Source: three-view drawing plus pictorial views. Frame: mm from the lowest corner of the part. A direction names the side the tool comes from. Give positions to 0.01 mm unless a question says otherwise; leave off trailing zeros. Loops run counter-clockwise (first coordinate to the right, second up) from the corner with the lowest first, then second, coordinate; pieces in that order, holes last.
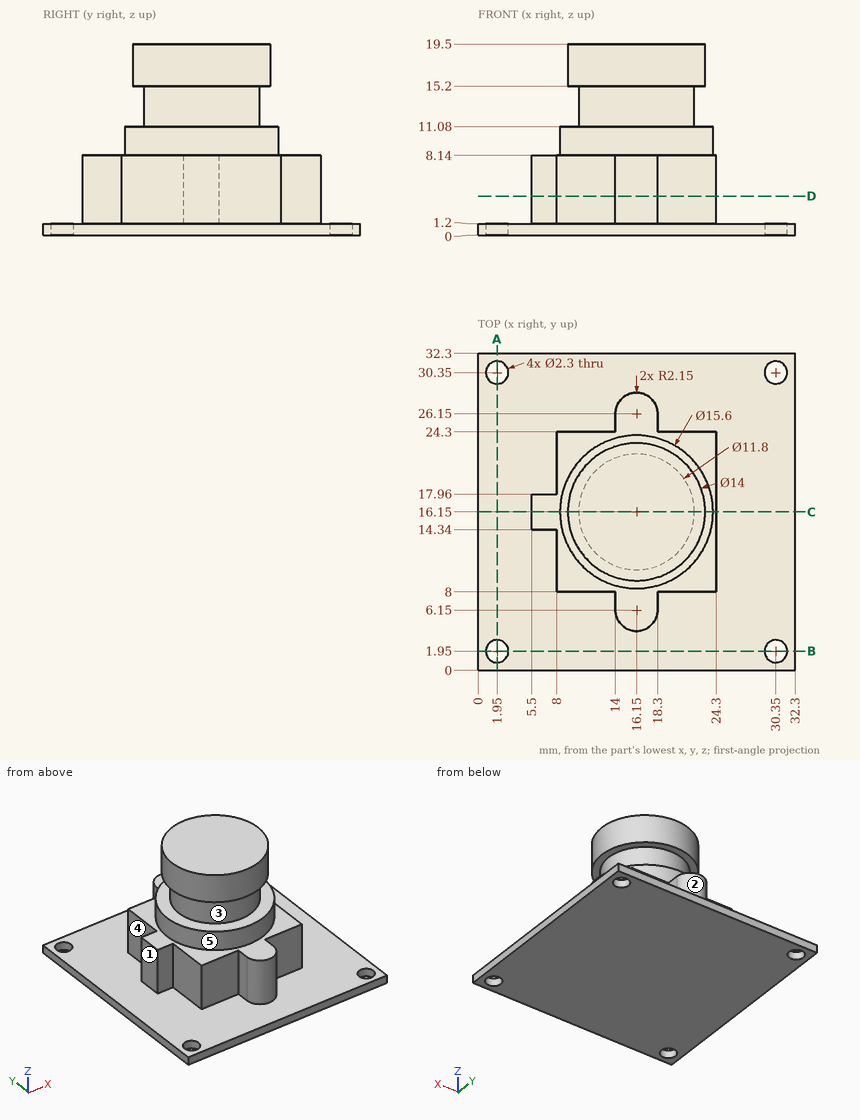
(1) Reachability of the marked faces 1, 2, 3, 4 and 5 from +Z, -Z, +X, -X, +Y, -Y: full face, straight path, thin tool, end or side. Return the list, or none.
Values follow:
face 1: +Z, -X, +Y, -Y
face 2: +Z, +Y
face 3: none
face 4: +Z, -X, +Y
face 5: +Z
(2) Cut plane A-A (x = 1.95). Return the cut outline in (y, z).
Values follow:
outline: (0, 0) - (0.8, 0) - (0.8, 1.2) - (0, 1.2) - close; (3.1, 0) - (29.2, 0) - (29.2, 1.2) - (3.1, 1.2) - close; (31.5, 0) - (32.3, 0) - (32.3, 1.2) - (31.5, 1.2) - close
(3) Pin query (flat end, axial travel): pin 1 Ø6.5 at (x, z) = (21, 5.5) entering from -Y; pin 2 Ø1 at (x, y) = (21.5, 5) entering from +Z; pin 3 Ø1.4 at (x, y) = (1.95, 30.35) entering from +Z; pin 4 Ø2 at (y, z) = (15, 4) entering from +X. Return the tip coordinate at first contact, or that it passes through.
Values follow:
pin 1: stops at y = 4.71
pin 2: stops at z = 1.2
pin 3: passes through
pin 4: stops at x = 24.3
(4) Ray query, probe 1 along Y at (x, z) = (1.95, 0.75); probe 2 along Z at (x, y) = (30.5, 5.5). Return the intervals inside material, ascending.
Values follow:
probe 1: y = 0 to 0.8, 3.1 to 29.2, 31.5 to 32.3
probe 2: z = 0 to 1.2
(5) Cut plane D-D (z = 4). Return the cut outline in (x, y), and give its area (3 significant figures).
Values follow:
outline: (5.5, 14.34) - (8, 14.34) - (8, 8) - (14, 8) - (14, 6.15) arc R2.15 ccw to (18.3, 6.15) - (18.3, 8) - (24.3, 8) - (24.3, 24.3) - (18.3, 24.3) - (18.3, 26.15) arc R2.15 ccw to (14, 26.15) - (14, 24.3) - (8, 24.3) - (8, 17.96) - (5.5, 17.96) - close
area: 305 mm2
(6) Cut plane C-C (y = 16.15). Return the cut outline in (x, z).
Values follow:
outline: (0, 0) - (32.3, 0) - (32.3, 1.2) - (24.3, 1.2) - (24.3, 8.14) - (23.95, 8.14) - (23.95, 11.08) - (22.05, 11.08) - (22.05, 15.2) - (23.15, 15.2) - (23.15, 19.5) - (9.15, 19.5) - (9.15, 15.2) - (10.25, 15.2) - (10.25, 11.08) - (8.35, 11.08) - (8.35, 8.14) - (5.5, 8.14) - (5.5, 1.2) - (0, 1.2) - close
